The listing builds one solid part. Answer for the finished solid, in the listing's coordinates (mm). A direction names the side the tool comes from. Give positions to 0.01 mm unless a question says otherwise; leave off trailing zeros. Write each loop counter-clockwise with the first axis right and the second up, starting at its lowest first coordinate (ties: lowest second). Pieces come first, ordered by that corner, then holes. Notation, with made-up numbers: (30.5, 86) - (79.5, 86) arc R29 ccw to (79.5, 111) - close; hole circle Ø4 at (9.25, 60.5). An arc over 180 degrees is marked (long way). One line per item, written item: value. Start each with the question number.
from build123d import *

# Parameters (mm, degrees)
SKETCH1_R                                            = 21.4
BOSS_EXTRUDE1_DEPTH                                  = 2
SKETCH2_R                                            = 6.5
BOSS_EXTRUDE2_DEPTH                                  = 4.7
SKETCH3_R                                            = 4
BOSS_EXTRUDE3_DEPTH                                  = 4.5
SKETCH5_R                                            = 3.25
CUT_EXTRUDE2_DEPTH                                   = 5.2
CUT_EXTRUDE1_REACH                                   = 13.2
SKETCH4_R                                            = 1.5
SKETCH6_W                                            = 0.85
SKETCH6_H                                            = 1
SKETCH7_W                                            = 0.5
SKETCH7_H                                            = 5.5
CUT_EXTRUDE3_DEPTH                                   = 22.4
CUT_EXTRUDE3_DEPTH_BACK                              = 22.4
CUT_EXTRUDE4_DEPTH                                   = 0.7
F_2_0_2_DIAMETER_HOLE6_D                             = 2
FILLET2_R                                            = 1
F_2_3_2_3_DIAMETER_HOLE1_D                           = 2.3
F_2_0_2_DIAMETER_HOLE8_D                             = 2
F_2_5_2_5_DIAMETER_HOLE1_D                           = 2.5
F_1_0_1_DIAMETER_HOLE1_D                             = 1
F_1_7_1_7_DIAMETER_HOLE2_D                           = 1.7
M1_4X0_3_TAPPED_HOLE1_D                              = 1.1
M2_TAPPED_HOLE1_D                                    = 1.6
CBORE_FOR_M1_7_HEX_SOCKET_HEAD_CAP_SCREW_D           = 1.5
CBORE_FOR_M1_7_HEX_SOCKET_HEAD_CAP_SCREW_CBORE_D     = 1.8
CBORE_FOR_M1_7_HEX_SOCKET_HEAD_CAP_SCREW_CBORE_DEPTH = 0.5
CBORE_FOR_M1_7_HEX_SOCKET_HEAD_CAP_S_2_D             = 1.5
CBORE_FOR_M1_7_HEX_SOCKET_HEAD_CAP_S_2_CBORE_D       = 1.8
CBORE_FOR_M1_7_HEX_SOCKET_HEAD_CAP_S_2_CBORE_DEPTH   = 1.2
CUT_EXTRUDE5_DEPTH                                   = 7.5
FILLET3_R                                            = 0.2
CHAMFER1_SIZE                                        = 0.2


with BuildPart() as part:
    # Sketch1 → Boss-Extrude1 (new body)
    with BuildSketch(Plane.XY):
        Circle(SKETCH1_R)
    extrude(amount=-BOSS_EXTRUDE1_DEPTH)

    # Sketch2 → Boss-Extrude2 (add)
    with BuildSketch(Plane(origin=(0, 0, -2), x_dir=(-1, 0, 0), z_dir=(0, 0, -1))):
        Circle(SKETCH2_R)
    extrude(amount=BOSS_EXTRUDE2_DEPTH)

    # Sketch3 → Boss-Extrude3 (add)
    with BuildSketch(Plane.XY):
        Circle(SKETCH3_R)
    extrude(amount=BOSS_EXTRUDE3_DEPTH)

    # Sketch5 → Cut-Extrude2 (cut)
    with BuildSketch(Plane(origin=(0, 0, -6.7), x_dir=(-1, 0, 0), z_dir=(0, 0, -1))):
        Circle(SKETCH5_R)
    extrude(amount=-CUT_EXTRUDE2_DEPTH, mode=Mode.SUBTRACT)

    # Sketch4 → Cut-Extrude1 (cut, up to next)
    with BuildSketch(Plane.XY.offset(4.5), mode=Mode.PRIVATE) as cut_extrude1_sk1:
        Circle(SKETCH4_R)
    cut_extrude1_tool1 = extrude(cut_extrude1_sk1.sketch, amount=-CUT_EXTRUDE1_REACH, mode=Mode.PRIVATE) & part.part
    add(cut_extrude1_tool1.solids().sort_by_distance((0, 0, 4.5))[0], mode=Mode.SUBTRACT)

    # Sketch6 → Cut-Revolve1 (revolve, cut)
    with BuildSketch(Plane(origin=(0, 0, 0), x_dir=(0, 0, -1), z_dir=(1, 0, 0))):
        with Locations((-1.225, 3.5)):
            Rectangle(SKETCH6_W, SKETCH6_H)
    revolve(axis=Axis((0, 0, 4.5), (0, 0, -1)), mode=Mode.SUBTRACT)

    # Sketch7 → Cut-Extrude3 (cut, two sides)
    with BuildSketch(Plane(origin=(0, 0, 0), x_dir=(0, 0, -1), z_dir=(1, 0, 0))) as cut_extrude3_sk:
        with Locations((6.45, 0)):
            Rectangle(SKETCH7_W, SKETCH7_H)
    extrude(amount=CUT_EXTRUDE3_DEPTH, mode=Mode.SUBTRACT)
    extrude(cut_extrude3_sk.sketch, amount=-CUT_EXTRUDE3_DEPTH_BACK, mode=Mode.SUBTRACT)

    # Sketch8 → Cut-Extrude4 (cut)
    with BuildSketch(Plane.XY):
        with BuildLine():
            Line((-2.6, 19), (3.4, 19))
            ThreePointArc((3.4, 19), (4.9, 17.5), (3.4, 16))
            Line((3.4, 16), (-2.6, 16))
            ThreePointArc((-2.6, 16), (-4.1, 17.5), (-2.6, 19))
        make_face()
    extrude(amount=-CUT_EXTRUDE4_DEPTH, mode=Mode.SUBTRACT)

    # Ø2.0 (2) Diameter Hole6 (through all)
    with Locations(Plane(origin=(0, 0, -2), x_dir=(1, 0, 0), z_dir=(0, 0, -1))):
        with Locations((-11.691342951, -6.75), (-8.677632731, -10.341599982), (-4.617271935, -12.685850381), (4.617271935, -12.685850381), (0, -13.5), (8.677632731, -10.341599982), (-12.685850381, 4.617271935), (-10.341599982, 8.677632731), (-6.75, 11.691342951), (2.344250399, 13.294904666), (6.75, 11.691342951), (10.341599982, 8.677632731), (12.685850381, 4.617271935), (13.5, 0), (12.685850381, -4.617271935), (-13.5, 0), (-2.344250399, 13.294904666)):
            Hole(F_2_0_2_DIAMETER_HOLE6_D / 2)

    # Fillet2
    fillet2_edges = [part.edges().sort_by_distance(p)[0] for p in [
        (6.5, 0, -2),
    ]]
    fillet(fillet2_edges, radius=FILLET2_R)

    # Ø2.3 (2.3) Diameter Hole1 (through all)
    with Locations(Plane(origin=(0, 0, -2), x_dir=(1, 0, 0), z_dir=(0, 0, -1))):
        with Locations((-19.5, 0), (-18.324006105, 6.669392795), (-14.937866641, 12.534358389), (-9.75, 16.887495374), (-3.386139465, 19.203751184), (3.386139465, 19.203751184), (9.75, 16.887495374), (14.937866641, 12.534358389)):
            Hole(F_2_3_2_3_DIAMETER_HOLE1_D / 2)

    # Ø2.0 (2) Diameter Hole8 (through all)
    with Locations(Plane(origin=(0, 0, -2), x_dir=(1, 0, 0), z_dir=(0, 0, -1))):
        with Locations((-17.616493237, -7.117525275), (12.713481521, -14.119751684), (17.616493237, 7.117525275)):
            Hole(F_2_0_2_DIAMETER_HOLE8_D / 2)

    # Ø2.5 (2.5) Diameter Hole1 (through all)
    with Locations(Plane(origin=(0, 0, -2), x_dir=(1, 0, 0), z_dir=(0, 0, -1))):
        with Locations((-5.871322893, -18.07007381)):
            Hole(F_2_5_2_5_DIAMETER_HOLE1_D / 2)

    # Ø1.0 (1) Diameter Hole1 (through all)
    with Locations(Plane(origin=(0, 0, -2), x_dir=(1, 0, 0), z_dir=(0, 0, -1))):
        with Locations((14.378193194, -2.535263394), (-11.18424887, -9.384699101)):
            Hole(F_1_0_1_DIAMETER_HOLE1_D / 2)

    # Ø1.7 (1.7) Diameter Hole2 (through all)
    with Locations(Plane(origin=(0, 0, -2), x_dir=(-1, 0, 0), z_dir=(0, 0, -1))):
        with Locations((13.5, 11.2)):
            Hole(F_1_7_1_7_DIAMETER_HOLE2_D / 2)

    # M1.4x0.3 Tapped Hole1 (through all)
    with Locations(Plane(origin=(0, 0, -2), x_dir=(1, 0, 0), z_dir=(0, 0, -1))):
        with Locations((-18.711347307, 3.299315376), (12.212964584, 14.554844419), (-12.212964584, 14.554844419), (0, 19)):
            Hole(M1_4X0_3_TAPPED_HOLE1_D / 2)

    # M2 Tapped Hole1 (through all)
    with Locations(Plane.XY):
        with Locations((6.498382723, 17.854159795), (-6.498382723, -17.854159795)):
            Hole(M2_TAPPED_HOLE1_D / 2)

    # CBORE for M1.7 Hex Socket Head Cap Screw (through all)
    with Locations(Plane.XY):
        with Locations((17.234135678, 3.038843109)):
            CounterBoreHole(CBORE_FOR_M1_7_HEX_SOCKET_HEAD_CAP_SCREW_D / 2, CBORE_FOR_M1_7_HEX_SOCKET_HEAD_CAP_SCREW_CBORE_D / 2, CBORE_FOR_M1_7_HEX_SOCKET_HEAD_CAP_SCREW_CBORE_DEPTH)

    # CBORE for M1.7 Hex Socket Head Cap S 2 (through all)
    with Locations(Plane(origin=(0, 0, -6.2), x_dir=(-1, 0, 0), z_dir=(0, 0, -1))):
        with Locations((-4.9, 0)):
            CounterBoreHole(CBORE_FOR_M1_7_HEX_SOCKET_HEAD_CAP_S_2_D / 2, CBORE_FOR_M1_7_HEX_SOCKET_HEAD_CAP_S_2_CBORE_D / 2, CBORE_FOR_M1_7_HEX_SOCKET_HEAD_CAP_S_2_CBORE_DEPTH)

    # Sketch41 → Cut-Extrude5 (cut, through all)
    with BuildSketch(Plane.XY.offset(-2)):
        with BuildLine():
            Line((-5.749818077, 19.314154426), (-6.135630169, 20.501561951))
            ThreePointArc((-6.135630169, 20.501561951), (-6.61296368, 20.352609449), (-7.086686686, 20.192544957))
            Line((-7.086686686, 20.192544957), (-6.700874593, 19.005137431))
            ThreePointArc((-6.700874593, 19.005137431), (-6.257594136, 19.258894455), (-5.749818077, 19.314154426))
        make_face()
    extrude(amount=CUT_EXTRUDE5_DEPTH, mode=Mode.SUBTRACT)

    # Fillet3
    fillet3_edges = [part.edges().sort_by_distance(p)[0] for p in [
        (-4, 0, 0),
    ]]
    fillet(fillet3_edges, radius=FILLET3_R)

    # Chamfer1
    chamfer1_edges = [part.edges().sort_by_distance(p)[0] for p in [
        (-4, 0, 4.5),
    ]]
    chamfer(chamfer1_edges, length=CHAMFER1_SIZE)


solid = part.part
Item 1: For faces 3 (the flat face through (-6.896, 19.607, -1.014)), 4 (the cylindrical face through (6.129, 17.144, -1.014)), 5 (the flat face through (3, -1, 0.8)), 6 (the cylindrical face through (4.9, 17.5, -0.3)), determine the directions among +Z, -Z, +X, -X, +Y, -Y from which every point of the face is accessible in a straight line to the end or side of a thin tool.
Item 2: The mould has two halves that part along X. Classify faces 1 (the flat face through (0, -4, -6.7)), 2 (the cylindrical face through (16.663, -7.418, -0.986)): +X half, -X half, draft (parallel to the pull), parting line (faces both ways), or undercut.
Item 3: Each of these flat-tipped pins is pushed along its axis until it touches: pin 1 Ø3 at (x, y) = (-17.62, 7.12) entering from +Z; pin 2 Ø1.4 at (x, y) = (-12.21, -14.55) entering from -Z; pin 3 Ø1.5 at (y, z) = (2, 2) entering from +X. Where does it stop, or does it pass through?
Item 4: Straight lines are drawn through the part: line 1 along Y through (x, z) = (0, -4.9); line 2 along Z through (x, y) = (2.5, 17); line 3 along Z through (x, y) = (2.5, -4.5). For each, find the intervals that lie inside material, in ascending order.
Item 5: Find section A-A on z = -3.5. Determine the outline of the cut face in (x, y).
Values:
1. face 3: +Z, -Z, +Y
1. face 4: +Z, -Z
1. face 5: none
1. face 6: +Z
2. face 1: draft
2. face 2: undercut
3. pin 1: z = 0
3. pin 2: z = -2
3. pin 3: x = 3.8
4. line 1: -6.5 to -3.25, 3.25 to 6.5
4. line 2: -2 to -0.7
4. line 3: -6.7 to 0
5. outline: circle Ø13 at (0, 0); hole circle Ø6.5 at (0, 0); hole circle Ø1.5 at (4.9, 0)
